```python
from build123d import *

# Parameters (mm, degrees)
BASE_EXTRUDE_DEPTH  = 12.7
BOSS_EXTRUDE1_DEPTH = 12.7


with BuildPart() as part:
    # Sketch1 → Base-Extrude (new, symmetric)
    with BuildSketch(Plane(origin=(0, 33.02, 0), x_dir=(1, 0, 0), z_dir=(0, 0, 1))):
        with BuildLine():
            Line((-20.6375, 24.13), (-20.6375, -9.6901))
            ThreePointArc((-20.6375, -9.6901), (-19.848914298, -11.593914298), (-17.9451, -12.3825))
            Line((-17.9451, -12.3825), (17.9451, -12.3825))
            ThreePointArc((17.9451, -12.3825), (19.848914298, -11.593914298), (20.6375, -9.6901))
            Line((20.6375, -9.6901), (20.6375, 24.13))
            ThreePointArc((20.6375, 24.13), (15.875, 28.8925), (11.1125, 24.13))
            Line((11.1125, 24.13), (11.1125, 23.09495))
            ThreePointArc((11.1125, 23.09495), (12.4587, 21.74875), (13.8049, 23.09495))
            Line((13.8049, 23.09495), (13.8049, 24.13))
            ThreePointArc((13.8049, 24.13), (15.875, 26.2001), (17.9451, 24.13))
            Line((17.9451, 24.13), (17.9451, -9.6901))
            Line((17.9451, -9.6901), (-17.9451, -9.6901))
            Line((-17.9451, -9.6901), (-17.9451, 24.13))
            ThreePointArc((-17.9451, 24.13), (-15.875, 26.2001), (-13.8049, 24.13))
            Line((-13.8049, 24.13), (-13.8049, 23.09495))
            ThreePointArc((-13.8049, 23.09495), (-12.4587, 21.74875), (-11.1125, 23.09495))
            Line((-11.1125, 23.09495), (-11.1125, 24.13))
            ThreePointArc((-11.1125, 24.13), (-15.875, 28.8925), (-20.6375, 24.13))
        make_face()
    base_extrude = extrude(amount=BASE_EXTRUDE_DEPTH, both=True)

    # Sketch2 → Boss-Extrude1 (add, symmetric)
    with BuildSketch(Plane.XY):
        with BuildLine():
            Line((-23.337499985, 50.8), (-23.337499985, 21.457899985))
            ThreePointArc((-23.337499985, 21.457899985), (-20.6375, 18.7579), (-23.337499985, 16.057900015))
            Line((-23.337499985, 16.057900015), (-23.337499985, -16.057900015))
            ThreePointArc((-23.337499985, -16.057900015), (-20.6375, -18.7579), (-23.337499985, -21.457899985))
            Line((-23.337499985, -21.457899985), (-23.337499985, -50.8))
            Line((-23.337499985, -50.8), (-20.6375, -50.8))
            Line((-20.6375, -50.8), (-20.6375, -23.434437154))
            ThreePointArc((-20.6375, -23.434437154), (-17.937500015, -18.7579), (-20.6375, -14.081362846))
            Line((-20.6375, -14.081362846), (-20.6375, 14.081362846))
            ThreePointArc((-20.6375, 14.081362846), (-17.937500015, 18.7579), (-20.6375, 23.434437154))
            Line((-20.6375, 23.434437154), (-20.6375, 50.8))
            Line((-20.6375, 50.8), (-23.337499985, 50.8))
        make_face()
    boss_extrude1 = extrude(amount=BOSS_EXTRUDE1_DEPTH, both=True)

    # Mirror1: Base-Extrude across plane
    add(base_extrude.mirror(Plane.ZX))

    # Mirror2: Boss-Extrude1 across plane
    add(boss_extrude1.mirror(Plane(origin=(0, 0, 0), x_dir=(0, 0, 1), z_dir=(1, 0, 0))))


solid = part.part
```
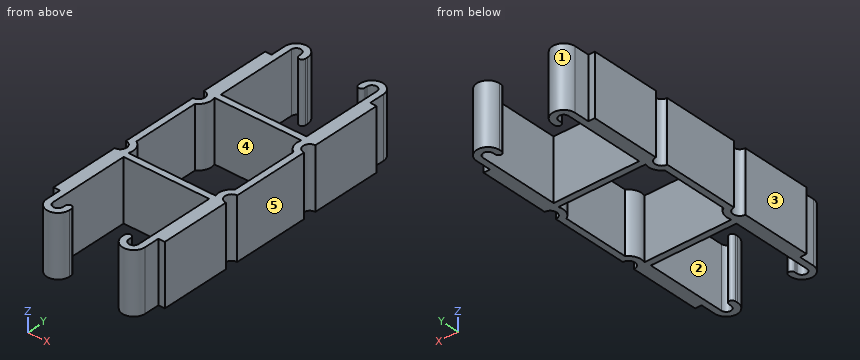
Input: part model. Units: mm. Frame: model coordinates. Face numbers are marked on the shaded views. A direction names the side the tool comes from. Round coordinates to 2 decimals unless told otherwise and drop trailing zeros. Loops run counter-clockwise (first coordinate to the right, second up) from the corner with the lowest first, then second, coordinate; pieces in that order, holes last.
1) Pin query (flat end, axial travel): pin 1 (4 mm diameter, centred on x = 2, z = -6.5, fed in from -Y); pin 2 (0.8 mm diameter, centred on y = 57, z = 5.5, fed in from -X); pin 3 (0.8 mm diameter, centred on y = -57, z = 5, fed in from +X). Return the tip coordinate at first contact, or that it passes through.
Ans:
pin 1: stops at y = -23.33
pin 2: stops at x = -20.64
pin 3: stops at x = 20.64
2) Section query A-A on x = 10. Return the cut outline in (y, z).
Ans:
outline: (-23.33, -12.7) - (-20.64, -12.7) - (-20.64, 12.7) - (-23.33, 12.7) - close; (20.64, -12.7) - (23.33, -12.7) - (23.33, 12.7) - (20.64, 12.7) - close
3) Material intervals for line 1 (X direction, y = 50, z = -10.5); line 2 (Y direction, x = 2.5, z = -7.5); line 3 (Y direction, x = -12, z = 3.5), sorted ascending.
Ans:
line 1: x = -23.34 to -17.95, 17.95 to 23.34
line 2: y = -23.33 to -20.64, 20.64 to 23.33
line 3: y = -59.92 to -54.85, -23.33 to -20.64, 20.64 to 23.33, 54.85 to 59.92
4) Set-up query: the marked faces 1 and 2. Return all of +Z, -Z, +X, -X, +Y, -Y with unobstructed straight access to the full face (end or side cutting, diameter ignored); none if empty.
Ans:
face 1: +Z, -Z, +Y
face 2: +Z, -Z
5) Section query B-B on y = 30. Return the cut outline in (x, z), plus the area to 3 significant figures.
Ans:
outline: (-23.34, -12.7) - (-17.95, -12.7) - (-17.95, 12.7) - (-23.34, 12.7) - close; (17.95, -12.7) - (23.34, -12.7) - (23.34, 12.7) - (17.95, 12.7) - close
area: 274 mm2
6) Pull-direction query (X, two-part tool) for the marked faces 3, 4 and 5; classes: released by +X, released by -X, zero draft, split by the parting line, or undercut.
Ans:
face 3: released by -X
face 4: undercut
face 5: released by +X
